Build history of the part. All positions in model axes, mm. Face numbers are marked on the shaded views. A direction names the side the tool comes from. Round coordinates to 2 decimals unless told otherwise and drop trailing zeros. Order: outer loops, then holes, each group sorted by start corner. A loop starts at its lowest first (then second) coordinate and runs counter-clockwise, first axis right, second up. Notation, with made-up numbers: (-4.5, 50.25) -> (22.5, 50.25) arc R14 ccw to (22.5, 68.25) -> close; hole circle Ø11 at (55, 0). An arc over 180 degrees is marked (long way). Use a Markdown table: item, result. Add a question column.
Item 1: Probe L1, parallel to Z at x = 4.5, y = 1.1; L2, parallel to Y at x = 67, z = 46; L3, parallel to Z at x = 43, y = 12.25. List the from-to ranges inside material, lowest first.
Item 2: Slice it at A-A, the plane z = 4.5. Give the cut face in (x, y), plus the area to 3 significant figures.
Item 3: Slice it at C-C, the plane x = 51.5. Give the cut face in (y, z).
Item 4: 3-axis set-ups, long thin cutter, end or side, ignore diameter. For the marked faces 1, 2 and 3: which of +Z, -Z, +X, -X, +Y, -Y reach the whole face in a straight line?
Item 5: Pin check, flat tips, straight feed: pin 1 (2.5 mm diameter, centred on x = 70.5, z = 4.5, fed in from +Y); pin 2 (2 mm diameter, centred on x = 60.5, y = -1.5, fed in from +Z); pin 3 (10 mm diameter, centred on y = 10, z = 95, fed in from +X); pin 4 (4.5 mm diameter, centred on y = 7.5, z = 97.5, fed in from -X). Stop position of each tip, or through.
Item 6: Slice it at B-B, the plane x = 4.5. Give the cut face in (y, z), plus the area to 3 significant figures.
Item 7: Slice it at D-D, the plane y = 12.5. Give the cut face in (x, z), plus the area to 3 significant figures.
from build123d import *

# Parameters (mm, degrees)
ESQUISSE1_W                   = 75
ESQUISSE1_H                   = 105
BOSS_EXTRU_1_DEPTH            = 1.7
DIAM_TRE_DU_PER_AGE_4_0_4_1_D = 4
CONG_1_R                      = 1
BOSS_EXTRU_2_DEPTH            = 12
BOSS_EXTRU_2_DEPTH_BACK       = 5
ESQUISSE4_W                   = 50
ESQUISSE4_H                   = 9


with BuildPart() as part:
    # Esquisse1 → Boss.-Extru.1 (new body)
    with BuildSketch(Plane(origin=(0, 0, 0), x_dir=(1, 0, 0), z_dir=(0, 1, 0))):
        with Locations((37.5, -52.5)):
            Rectangle(ESQUISSE1_W, ESQUISSE1_H)
    extrude(amount=BOSS_EXTRU_1_DEPTH)

    # Diamètre du perçage Ø4.0 (4)1 (through all)
    with Locations(Plane(origin=(0, 1.7, 0), x_dir=(1, 0, 0), z_dir=(0, 1, 0))):
        with Locations((70.5, -100.5), (4.5, -100.5), (70.5, -4.5), (4.5, -4.5)):
            Hole(DIAM_TRE_DU_PER_AGE_4_0_4_1_D / 2)

    # Congé1
    cong_1_edges = [part.edges().sort_by_distance(p)[0] for p in [
        (0, 0.85, 0),
        (75, 0.85, 0),
        (75, 0.85, 105),
        (0, 0.85, 105),
    ]]
    fillet(cong_1_edges, radius=CONG_1_R)

    # Esquisse4 → Boss.-Extru.2 (add, two sides: drawn at the far end of the back side and taken through both)
    with BuildSketch(Plane(origin=(0, 1.7, 0), x_dir=(1, 0, 0), z_dir=(0, 1, 0)).offset(-BOSS_EXTRU_2_DEPTH_BACK)):
        with Locations((37.5, -96)):
            Rectangle(ESQUISSE4_W, ESQUISSE4_H)
    extrude(amount=BOSS_EXTRU_2_DEPTH + BOSS_EXTRU_2_DEPTH_BACK)


solid = part.part
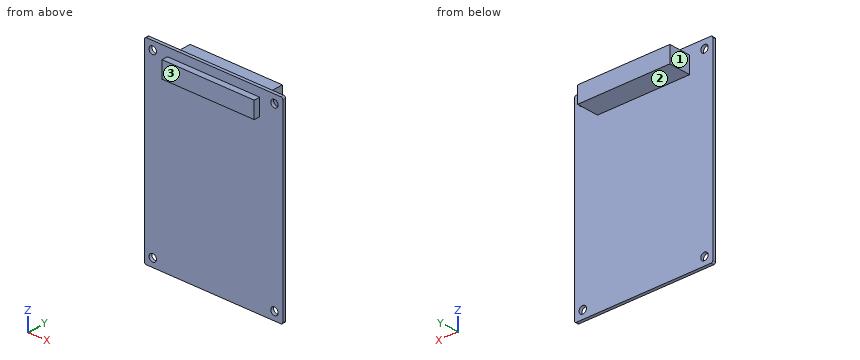
Check sheet entries:
| question | item | result |
|---|---|---|
| 1 | L1 | 0 to 2.5, 6.5 to 98.5, 102.5 to 105 |
| 1 | L2 | 0 to 1.7 |
| 1 | L3 | 91.5 to 100.5 |
| 2 | outline | (0, 0) -> (2.5, 0) -> (2.5, 1.7) -> (0, 1.7) -> close; (6.5, 0) -> (68.5, 0) -> (68.5, 1.7) -> (6.5, 1.7) -> close; (72.5, 0) -> (75, 0) -> (75, 1.7) -> (72.5, 1.7) -> close |
| 2 | area | 114 mm2 |
| 3 | outline | (-3.3, 91.5) -> (0, 91.5) -> (0, 0) -> (1.7, 0) -> (1.7, 91.5) -> (13.7, 91.5) -> (13.7, 100.5) -> (1.7, 100.5) -> (1.7, 105) -> (0, 105) -> (0, 100.5) -> (-3.3, 100.5) -> close |
| 4 | face 1 | +Z, -Z, -X, +Y |
| 4 | face 2 | -Z, +X, -X, +Y |
| 4 | face 3 | +Z, -Z, +X, -X, -Y |
| 5 | pin 1 | through |
| 5 | pin 2 | z = 100.5 |
| 5 | pin 3 | x = 62.5 |
| 5 | pin 4 | x = 12.5 |
| 6 | outline | (0, 0) -> (1.7, 0) -> (1.7, 2.5) -> (0, 2.5) -> close; (0, 6.5) -> (1.7, 6.5) -> (1.7, 98.5) -> (0, 98.5) -> close; (0, 102.5) -> (1.7, 102.5) -> (1.7, 105) -> (0, 105) -> close |
| 6 | area | 165 mm2 |
| 7 | outline | (12.5, 91.5) -> (62.5, 91.5) -> (62.5, 100.5) -> (12.5, 100.5) -> close |
| 7 | area | 450 mm2 |
